Source: CAD feature listing. Evaluate the final solid. Frame: model axes, mm. Face numbers are marked on the shaded views. A direction names the side the tool comes from. Round coordinates to 2 decimals unless told otherwise and drop trailing zeros. Order: outer loops, then holes, each group sorted by start corner. A loop starts at its lowest first (then second) coordinate and runs counter-clockwise, first axis right, second up. Notation, with made-up numbers: (58, -8.5) - (108, -8.5) arc R26 cw to (108, 20.5) - close; hole circle Ø8 at (41.5, 68). An arc over 180 degrees is marked (long way). Use one line per item in the form item = value. Start each with the question number.
Q1. Set-up query: the marked faces 4, 5, 6 and 7. Return all of +Z, -Z, +X, -X, +Y, -Y with unobstructed straight access to the full face (end or side cutting, diameter ignored); none if empty.
Q2. Cut plane B-B, the plane x = 44. Return the cut outline in (y, z), and give its area (3 significant figures).
Q3. Cut plane A-A, the plane y = 18.5. Give the number of separate pieces and of enclosed holes in the cut face, and give its area (3 significant figures).
Q4. Draft query along X for the marked faces 1, 2 and 3. Return one class per face: released by +X, released by -X, zero draft, split by the parting line, or undercut.
Q5. Pin query (flat end, axial travel): pin 1 Ø1 at (y, z) = (8.5, 47.5) entering from -X; pin 2 Ø3 at (x, y) = (-72.5, -18.5) entering from -Z; pin 3 Ø2 at (y, z) = (-3.5, 38.5) entering from -X. Return the tip coordinate at first contact, or that it passes through.
Q6. Ray query, line 1 (X direction, y = 20, z = 5.5); line 2 (X direction, y = -12.5, z = 5); line 3 (Y direction, x = 2.5, z = -25). Return the intervals inside material, ascending. Write a range as [from, to].
from build123d import *

# Parameters (mm, degrees)
F0_R     = 22.225
F1_DEPTH = 12.7
F0_R_2   = 9.525
F0_R_3   = 14.2875
F2_DEPTH = 22.225


with BuildPart() as f1:
    # F0 (on Front) → F1 (new body, symmetric)
    with BuildSketch(Plane.XZ):
        with BuildLine():
            ThreePointArc((-39.064243, 52.658537), (-54.841462, 28.445004), (-82.171843, 19.05))
            Line((-82.171843, 19.05), (-63.2968, 19.05))
            ThreePointArc((-63.2968, 19.05), (-44.2468, 0), (-63.2968, -19.05))
            Line((-63.2968, -19.05), (-88.6968, -19.05))
            Line((-88.6968, -19.05), (-3.164031, -41.261841))
            ThreePointArc((-3.164031, -41.261841), (16.376083, -40.683694), (32.544555, -29.695938))
            ThreePointArc((32.544555, -29.695938), (41.583612, -19.519195), (55.183261, -20.085065))
            ThreePointArc((55.183261, -20.085065), (72.465036, -15.685246), (80.9498, 0))
            ThreePointArc((80.9498, 0), (76.06793, 27.686462), (62.011144, 52.033528))
            ThreePointArc((62.011144, 52.033528), (44.80973, 59.971876), (27.736253, 51.761978))
            ThreePointArc((27.736253, 51.761978), (12.908055, 45.3375), (0.133292, 55.234711))
            ThreePointArc((0.133292, 55.234711), (1.220688, 51.498707), (1.5875, 47.625))
            ThreePointArc((1.5875, 47.625), (-21.585988, 27.143907), (-39.064243, 52.658537))
        make_face()
        Circle(F0_R, mode=Mode.SUBTRACT)
        with BuildLine():
            ThreePointArc((69.85, 0), (58.7248, -11.1252), (47.5996, 0))
            ThreePointArc((47.5996, 0), (44.728993, 16.280022), (36.463409, 30.596433))
            ThreePointArc((36.463409, 30.596433), (37.834666, 46.269971), (53.508204, 44.898715))
            ThreePointArc((53.508204, 44.898715), (65.63753, 23.890107), (69.85, 0))
        make_face(mode=Mode.SUBTRACT)
    extrude(amount=F1_DEPTH, both=True)

    # F0 (on Front) → F2 (join, symmetric)
    with BuildSketch(Plane.XZ):
        with BuildLine():
            ThreePointArc((0.133292, 55.234711), (-20.403436, 68.218072), (-39.064243, 52.658537))
            ThreePointArc((-39.064243, 52.658537), (-21.585988, 27.143907), (1.5875, 47.625))
            ThreePointArc((1.5875, 47.625), (1.220688, 51.498707), (0.133292, 55.234711))
        make_face()
        with Locations((-19.05, 47.625)):
            Circle(F0_R_2, mode=Mode.SUBTRACT)
        with BuildLine():
            Line((-82.171843, 19.05), (-88.6968, 19.05))
            ThreePointArc((-88.6968, 19.05), (-107.7468, 0), (-88.6968, -19.05))
            Line((-88.6968, -19.05), (-63.2968, -19.05))
            ThreePointArc((-63.2968, -19.05), (-44.2468, 0), (-63.2968, 19.05))
            Line((-63.2968, 19.05), (-82.171843, 19.05))
        make_face()
        with BuildLine():
            ThreePointArc((-88.6968, -11.0998), (-99.7966, 0), (-88.6968, 11.0998))
            Line((-88.6968, 11.0998), (-63.2968, 11.0998))
            ThreePointArc((-63.2968, 11.0998), (-52.197, 0), (-63.2968, -11.0998))
            Line((-63.2968, -11.0998), (-88.6968, -11.0998))
        make_face(mode=Mode.SUBTRACT)
        Circle(F0_R)
        Circle(F0_R_3, mode=Mode.SUBTRACT)
    extrude(amount=F2_DEPTH, both=True)


solid = f1.part
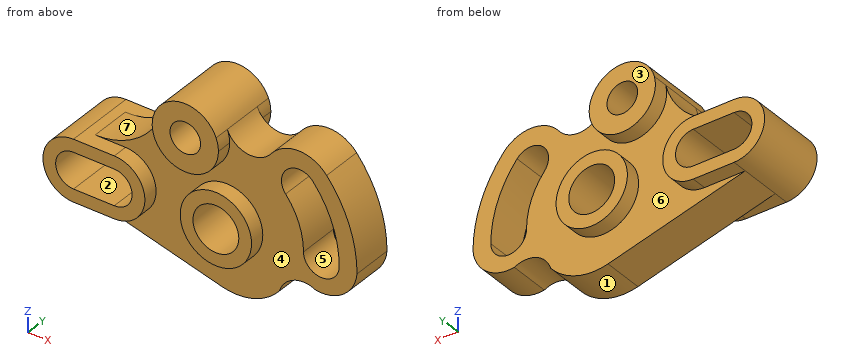
Completed:
q1.face_4 = -Y
q1.face_5 = +Y, -Y
q1.face_6 = +Y
q1.face_7 = +Z, -X, +Y, -Y
q2.outline = (-12.7, -18.72) - (12.7, -18.72) - (12.7, 18.16) - (-12.7, 18.16) - close; (-12.7, 48.83) - (12.7, 48.83) - (12.7, 59.95) - (-12.7, 59.95) - close
q2.area = 1,220 mm2
q3.separate_pieces = 3
q3.enclosed_holes = 3
q3.area = 3,120 mm2
q4.face_1 = split by the parting line
q4.face_2 = undercut
q4.face_3 = zero draft
q5.pin_1 = -40.9
q5.pin_2 = -19.05
q5.pin_3 = -46.12
q6.line_1 = [-106.94, -98.34], [-53.66, -45.06], [-21.53, -13.19], [13.19, 21.53]
q6.line_2 = [-107.08, -98.61], [-53.39, -13.38], [13.38, 47.34], [69.67, 80.8]
q6.line_3 = [-12.7, 12.7]
